```python
from build123d import *

# Parameters (mm, degrees)
SKETCH2_R               = 21
BOSS_EXTRUDE1_DEPTH     = 35
SKETCH3_W               = 42
SKETCH3_H               = 42
BOSS_EXTRUDE2_DEPTH     = 20
CHAMFER1_SIZE           = 5
CUT_EXTRUDE1_DEPTH      = 20
CUT_EXTRUDE1_DEPTH_BACK = 46.90206967
SKETCH4_R               = 1.5
CUT_EXTRUDE2_START      = 2
CUT_EXTRUDE2_DEPTH      = 15
SKETCH6_R               = 2.75
CUT_EXTRUDE3_DEPTH      = 63.505999712
SKETCH8_R               = 2
CUT_EXTRUDE4_DEPTH      = 8
BOSS_EXTRUDE3_START     = 2
SKETCH9_R               = 9.628132553
SKETCH9_R_2             = 2.75
BOSS_EXTRUDE3_DEPTH     = 2


with BuildPart() as part:
    # Sketch2 → Boss-Extrude1 (new body)
    with BuildSketch(Plane.XY):
        Circle(SKETCH2_R)
    extrude(amount=BOSS_EXTRUDE1_DEPTH)

    # Sketch3 → Boss-Extrude2 (add)
    with BuildSketch(Plane.XY.offset(35)):
        Rectangle(SKETCH3_W, SKETCH3_H)
    extrude(amount=BOSS_EXTRUDE2_DEPTH)

    # Chamfer1
    chamfer1_edges = [part.edges().sort_by_distance(p)[0] for p in [
        (-21, -21, 45),
        (21, -21, 45),
        (21, 21, 45),
        (-21, 21, 45),
    ]]
    chamfer(chamfer1_edges, length=CHAMFER1_SIZE)

    # Sketch4 → Cut-Extrude1 (cut, two sides: drawn at the far end of the back side and taken through both)
    with BuildSketch(Plane(origin=(0, 0, 35), x_dir=(-1, 0, 0), z_dir=(0, 0, -1)).offset(-CUT_EXTRUDE1_DEPTH_BACK)):
        with Locations(Location((15.5, 15.5, 0), (0, 0, 174.410746944))):
            Circle(SKETCH4_R)
        with Locations(Location((-15.5, 15.5, 0), (0, 0, 180))):
            Circle(SKETCH4_R)
        with Locations(Location((15.5, -15.5, 0), (0, 0, 180))):
            Circle(SKETCH4_R)
        with Locations(Location((-15.5, -15.5, 0), (0, 0, 95.589253056))):
            Circle(SKETCH4_R)
    extrude(amount=CUT_EXTRUDE1_DEPTH + CUT_EXTRUDE1_DEPTH_BACK, mode=Mode.SUBTRACT)

    # Sketch5 → Cut-Extrude2 (cut)
    with BuildSketch(Plane(origin=(0, 0, 35), x_dir=(-1, 0, 0), z_dir=(0, 0, -1)).offset(CUT_EXTRUDE2_START)):
        with BuildLine():
            Line((15.843578324, 13.843578324), (23.156421676, 13.843578324))
            Line((23.156421676, 13.843578324), (23.156421676, 23.156421676))
            Line((23.156421676, 23.156421676), (13.843578324, 23.156421676))
            Line((13.843578324, 23.156421676), (13.843578324, 15.843578324))
            ThreePointArc((13.843578324, 15.843578324), (14.429364762, 14.429364762), (15.843578324, 13.843578324))
        make_face()
        with BuildLine():
            Line((23.156421676, -13.843578324), (23.156421676, -23.156421676))
            Line((23.156421676, -23.156421676), (13.843578324, -23.156421676))
            Line((13.843578324, -23.156421676), (13.843578324, -15.843578324))
            ThreePointArc((13.843578324, -15.843578324), (14.429364762, -14.429364762), (15.843578324, -13.843578324))
            Line((15.843578324, -13.843578324), (23.156421676, -13.843578324))
        make_face()
        with BuildLine():
            Line((-23.156421676, 13.843578324), (-23.156421676, 23.156421676))
            Line((-23.156421676, 23.156421676), (-13.843578324, 23.156421676))
            Line((-13.843578324, 23.156421676), (-13.843578324, 15.843578324))
            ThreePointArc((-13.843578324, 15.843578324), (-14.429364762, 14.429364762), (-15.843578324, 13.843578324))
            Line((-15.843578324, 13.843578324), (-23.156421676, 13.843578324))
        make_face()
        with BuildLine():
            Line((-15.843578324, -13.843578324), (-23.156421676, -13.843578324))
            Line((-23.156421676, -13.843578324), (-23.156421676, -23.156421676))
            Line((-23.156421676, -23.156421676), (-13.843578324, -23.156421676))
            Line((-13.843578324, -23.156421676), (-13.843578324, -15.843578324))
            ThreePointArc((-13.843578324, -15.843578324), (-14.429364762, -14.429364762), (-15.843578324, -13.843578324))
        make_face()
    extrude(amount=-CUT_EXTRUDE2_DEPTH, mode=Mode.SUBTRACT)

    # Sketch6 → Cut-Extrude3 (cut, through all)
    with BuildSketch(Plane(origin=(0, 0, 0), x_dir=(-1, 0, 0), z_dir=(0, 0, -1))):
        Circle(SKETCH6_R)
    extrude(amount=-CUT_EXTRUDE3_DEPTH, mode=Mode.SUBTRACT)

    # Sketch8 → Cut-Extrude4 (cut)
    with BuildSketch(Plane(origin=(0, 0, 0), x_dir=(-1, 0, 0), z_dir=(0, 0, -1))):
        with Locations((0, 17.5)):
            Circle(SKETCH8_R)
        with Locations((17.5, 0)):
            Circle(SKETCH8_R)
        with Locations((0, -17.5)):
            Circle(SKETCH8_R)
        with Locations((-17.5, 0)):
            Circle(SKETCH8_R)
    extrude(amount=-CUT_EXTRUDE4_DEPTH, mode=Mode.SUBTRACT)

    # Sketch9 → Boss-Extrude3 (add)
    with BuildSketch(Plane(origin=(0, 0, 0), x_dir=(-1, 0, 0), z_dir=(0, 0, -1)).offset(BOSS_EXTRUDE3_START)):
        with Locations(Location((0, 0, 0), (0, 0, 180))):
            Circle(SKETCH9_R)
        Circle(SKETCH9_R_2, mode=Mode.SUBTRACT)
    extrude(amount=-BOSS_EXTRUDE3_DEPTH)


solid = part.part
```
Geometry check sheet. Reference: the model listing, model coordinates, mm. A direction names the side the tool comes from. Coordinates: 2 decimals unless noted, no trailing zeros. Order: outer loops, then holes, each group sorted by start corner. A loop starts at its lowest first (then second) coordinate and runs counter-clockwise, first axis right, second up. Notation, with made-up numbers: M 64,-2.75 L 72,-2.75 A32 cw 72,29.25 Z; hole C -27.5,89.5 d11. An arc over 180 degrees is marked long. One line per question, with ' | ' between items. Start each with the question number.
Item 1: Cross-section at C-C on x = -10.5. Enter the section's corners in (y, z).
Item 2: Cross-section at B-B on y = 5. Enter the section's corners in (x, z), then the cut area to 3 significant figures.
Item 3: Gauge pin test, flat ends, axial feed: pin 1 (3 mm diameter, centred on y = 15, z = 47.5, fed in from -X); pin 2 (12 mm diameter, centred on x = -8, z = 13.5, fed in from +Y); pin 3 (4 mm diameter, centred on x = 18.5, y = -5.5, fed in from -Z); pin 4 (6 mm diameter, centred on y = -6.5, z = 23, fed in from -X). Record the tip position at first contact, or that the pin passes through.
Item 4: Cross-section at A-A on z = 46.5. Enter the section's corners in (x, y), then the cut area to 3 significant figures.
Item 5: Set-up check for faces 1 (the flat face through (18, 13.844, 41)), 2 (the cylindrical face through (-14.41, -14.45, 40.39)), 3 (the cylindrical face through (15.063, -14.065, 51.549)), 4 (the flat face through (9, -4, 0)): record each of +Z, -Z, +X, -X, +Y, -Y from which the full face is reachable in a straight line by a thin tool's end or side.
Item 6: Material ranges on L1, parallel to Y at x = -15.5, z = 51.5; L2, parallel to Y at x = 0, z = 42.5; L3, parallel to X at y = -15, z = 52, recorded low to high. Write a range as [from, to].
Item 7: Cross-section at D-D on x = 7.5. Enter the section's corners in (y, z).
Item 8: Draft check along Y on faces 5 (the cylindrical face through (14, 15.43, 51.55)), 6 (the flat face through (-18, 13.844, 41)), 7 (the flat face through (13.844, 18, 41)). Enter one of: pulls with the +Y half, pulls with the -Y half, needs draft (parallel to the pull), parting line crosses it, or undercut.
Findings:
1) outline: M -21,35 L -18.19,35 L -18.19,0 L 18.19,0 L 18.19,35 L 21,35 L 21,55 L -21,55 Z
2) outline: M -21,35 L -20.4,35 L -20.4,0 L -8.23,0 L -8.23,-2 L 8.23,-2 L 8.23,0 L 20.4,0 L 20.4,35 L 21,35 L 21,55 L -21,55 Z | area: 2,300 mm²
3) pin 1: stops at x = -21 | pin 2: stops at y = 20.9 | pin 3: stops at z = 0 | pin 4: stops at x = -20.71
4) outline: M -21,-13.84 L -15.84,-13.84 A2 cw -13.84,-15.84 L -13.84,-21 L 13.84,-21 L 13.84,-15.84 A2 cw 15.84,-13.84 L 21,-13.84 L 21,13.84 L 15.84,13.84 A2 cw 13.84,15.84 L 13.84,21 L -13.84,21 L -13.84,15.84 A2 cw -15.84,13.84 L -21,13.84 Z; hole C 0,0 d5.5 | area: 1,540 mm²
5) face 1: -Z, +X, +Y | face 2: -X, -Y | face 3: +Z | face 4: -Z
6) L1: y = [-21, -17], [-14, 14], [17, 21] | L2: y = [-21, -2.75], [2.75, 21] | L3: x = [-21, -16.91], [-14.09, 14.09], [16.91, 21]
7) outline: M -21,35 L -19.62,35 L -19.62,0 L -6.04,0 L -6.04,-2 L 6.04,-2 L 6.04,0 L 19.62,0 L 19.62,35 L 21,35 L 21,55 L -21,55 Z
8) face 5: undercut | face 6: pulls with the +Y half | face 7: needs draft
